```python
from build123d import *

# Parameters (mm, degrees)
ESQUISSE2_R      = 2.5
EXTRUSION1_DEPTH = 10
CONG_1_R         = 1
CHANFREIN1_SIZE  = 0.5
CONG_2_R         = 0.5


with BuildPart() as part:
    # Esquisse1 → Révolution1 (revolve)
    with BuildSketch(Plane.XY):
        with BuildLine():
            Line((0, 17), (10, 17))
            Line((10, 17), (10, 0))
            Line((10, 0), (5.338539126, 0))
            ThreePointArc((5.338539126, 0), (5.448623679, 6.311862178), (0, 9.5))
            Line((0, 9.5), (0, 17))
        make_face()
    revolve(axis=Axis((0, 0, 0), (0, 1, 0)))

    # Esquisse2 → Extrusion1 (add)
    with BuildSketch(Plane(origin=(0, 17, 0), x_dir=(1, 0, 0), z_dir=(0, 1, 0))):
        Circle(ESQUISSE2_R)
    extrude(amount=EXTRUSION1_DEPTH)

    # Congé1
    cong_1_edges = [part.edges().sort_by_distance(p)[0] for p in [
        (-10, 0, 0),
    ]]
    fillet(cong_1_edges, radius=CONG_1_R)

    # Chanfrein1
    chanfrein1_edges = [part.edges().sort_by_distance(p)[0] for p in [
        (-2.5, 27, 0),
    ]]
    chamfer(chanfrein1_edges, length=CHANFREIN1_SIZE)

    # Congé2
    cong_2_edges = [part.edges().sort_by_distance(p)[0] for p in [
        (-2.5, 17, 0),
    ]]
    fillet(cong_2_edges, radius=CONG_2_R)


solid = part.part
```
Source: CAD feature listing. Evaluate the final solid. Frame: model axes, mm. A direction names the side the tool comes from. Coordinates: 2 decimals unless noted, no trailing zeros. Loops run counter-clockwise (first coordinate to the right, second up) from the corner with the lowest first, then second, coordinate; pieces in that order, holes last. Notation, with made-up numbers: (72, 52) - (103, 52) arc R18 cw to (103, 87) - close; hole circle Ø6 at (78, -29). An arc over 180 degrees is marked (long way). Answer as CSV lines item,"result".
1. Contact query for flat-ended pins moving along their axis: pin 1 (6 mm diameter, centred on x = 2, z = -5, fed in from +Y); pin 2 (5 mm diameter, centred on y = 9, z = -5, fed in from -X); pin 3 (2 mm diameter, centred on x = -6.5, y = 15, fed in from +Z). Output: stop coordinate, or through.
Established:
pin 1,"stops at y = 26.61"
pin 2,"stops at x = -9.68"
pin 3,"stops at z = 8.35"
2. Section C-C (y = 13.25). Return loops of the section in (x, z), then the cut area to 3 significant figures.
Established:
outline,"circle Ø20 at (0, 0)"
area,"314 mm2"
3. Section D-D (y = 19). Return loops of the section in (x, z).
Established:
outline,"circle Ø5 at (0, 0)"
4. Section B-B (x = 0). Return loops of the section in (y, z), then the cut area to 3 significant figures.
Established:
outline,"(0, -9) arc R1 ccw to (1, -10) - (17, -10) - (17, -3) arc R0.5 cw to (17.5, -2.5) - (26.5, -2.5) - (27, -2) - (27, 2) - (26.5, 2.5) - (17.5, 2.5) arc R0.5 cw to (17, 3) - (17, 10) - (1, 10) arc R1 ccw to (0, 9) - (0, 5.34) arc R6.25 cw (long way) to (0, -5.34) - close"
area,"289 mm2"
5. Ray query, line 1 (Y direction, x = 3, z = -7.75); line 2 (Z direction, x = -2.25, y = 1.75); line 3 (X direction, y = 5.25, z = 0.25). Return the intervals inside material, ascending.
Established:
line 1,"y = 0 to 17"
line 2,"z = -9.74 to -5.63, 5.63 to 9.74"
line 3,"x = -10 to -5.92, 5.92 to 10"
6. Reachability of faces 1 (the flat face through (-2.1, 17, -2.4)), 2 (the flat face through (0, 27, 0)) from +Z, -Z, +X, -X, +Y, -Y: full face, straight path, thin tool, end or side. Return the list, or none.
Established:
face 1,"+Y"
face 2,"+Z, -Z, +X, -X, +Y"
7. Section A-A (z = 0). Return loops of the section in (x, y).
Established:
outline,"(-10, 1) arc R1 ccw to (-9, 0) - (-5.34, 0) arc R6.25 cw (long way) to (5.34, 0) - (9, 0) arc R1 ccw to (10, 1) - (10, 17) - (3, 17) arc R0.5 cw to (2.5, 17.5) - (2.5, 26.5) - (2, 27) - (-2, 27) - (-2.5, 26.5) - (-2.5, 17.5) arc R0.5 cw to (-3, 17) - (-10, 17) - close"
